Design review of the part built by this model. Coordinates are the model's own, in mm. A direction names the side the tool comes from. Coordinates: 2 decimals unless noted, no trailing zeros. Order: outer loops, then holes, each group sorted by start corner. A loop starts at its lowest first (then second) coordinate and runs counter-clockwise, first axis right, second up.
Autodesk Inventor part; units mm, degrees
ref_plane "YZ Plane" through (0, 0, 0) normal (1, 0, 0) x (0, 1, 0)
ref_plane "XZ Plane" through (0, 0, 0) normal (0, 1, 0) x (-1, 0, 0)
ref_plane "XY Plane" through (0, 0, 0) normal (0, 0, 1) x (1, 0, 0)
sketch "Sketch1" plane through (0, 0, 0) normal (0, 1, 0) x (-1, 0, 0)
  line L0 (-52.0419, 20) -> (-52.0419, -20)
  line L1 (52.0419, 20) -> (-52.0419, -20) construction
  line L2 (-52.0419, 20) -> (52.0419, -20) construction
  line L3 (305.5497, 112) -> (270.3665, 112)
  line L4 (270.3665, -112) -> (305.5497, -112)
  line L5 (305.5497, -112) -> (305.5497, 112)
  line L6 (305.5497, 112) -> (270.3665, -112) construction
  line L7 (270.3665, 112) -> (305.5497, -112) construction
  line L8 (270.3665, 20) -> (-52.0419, 20)
  line L9 (270.3665, 112) -> (270.3665, 20)
  line L10 (270.3665, -20) -> (270.3665, -112)
  line L11 (-52.0419, -20) -> (270.3665, -20)
  point P0 (0, 0)
  point P1 (287.9581, 0)
  point P2 (-52.0419, 0)
  dimension "d17" = 224
  dimension "d19" = 40
  dimension "d20" = 340
extrude "Extrusion1" add sketch "Sketch1" along normal blind 34
sketch "Sketch2" plane through (-305.5497, 0, 112) normal (0, 0, 1) x (1, 0, 0)
  circle A0 centre (17.5916, 16) radius 4.25
  line L0 (0, 0) -> (35.1832, 0)
  line L1 (0, 0) -> (0, 34)
  point P0 (305.5497, 0)
  point P1 (17.5916, 0)
  dimension "d2" = 8.5
  dimension "d3" = 16
sketch "Sketch3" plane through (52.0419, 0, 20) normal (1, 0, 0) x (0, 0, -1)
  circle A0 centre (20, 16) radius 4.25
  line L0 (0, 0) -> (40, 0)
  line L1 (40, 0) -> (40, 34)
  point P0 (20, 0)
  point P1 (20, 0)
  dimension "d4" = 8.5
  dimension "d5" = 16
sketch "Sketch4" plane through (-270.3665, 0, -112) normal (0, 0, -1) x (-1, 0, 0)
  circle A0 centre (17.5916, 16) radius 4.25
  line L0 (0, 0) -> (35.1832, 0)
  line L1 (0, 0) -> (0, 34)
  point P0 (-270.3665, 0)
  point P1 (17.5916, 0)
  dimension "d6" = 8.5
  dimension "d7" = 16
extrude "Extrusion2" cut sketch "Sketch4" against normal blind 10
extrude "Extrusion3" cut sketch "Sketch2" against normal blind 10
extrude "Extrusion4" cut sketch "Sketch3" against normal blind 10
properties part number "T"
1. For faces 4 (the cylindrical face through (47.11, 11.85, 0.92)), 5 (the flat face through (-111, 17, 20)), 6 (the cylindrical face through (-292.204, 16.187, 107.07)), list the 3-axis set-ups (+Z, -Z, +X, -X, +Y, -Y) from which the entire face can be reached by the end or side of a thin tool; tool diameter is ignored.
2. Add section B-B (z = -38.5). Give the boundary of the cut face in (x, y), and give its area (3 significant figures).
3. Insertion check: pin 1 (4 mm diameter, centred on x = -122, y = 24, fed in from +Z); pin 2 (17 mm diameter, centred on y = 9, z = -53, fed in from +X); pin 3 (10 mm diameter, centred on x = -117, y = 23.5, fed in from -Z). Each pin has a flat end and moves straight along its axis. Give the tip position at first contact, or say it passes through.
4. Add section A-A (y = 16). Give the boundary of the cut face in (x, z), and give its area (3 significant figures).
5. To check wall thickness, follow line 1 (Y direction, x = 46, z = 0); line 2 (Z direction, x = -9.5, y = 23); line 3 (X direction, y = 5, z = -80). State the ranges of each line that lie inside material, in increasing order.
6. Mouldability with a two-part tool opening along X and no side actions: class faces 1 (the flat face through (-107, 17, -20)), 2 (the flat face through (-288, 16, 102)), 3 (the flat face through (-270.366, 17, 67)) as pulls with the +X half, pulls with the -X half, needs draft (parallel to the pull), parting line crosses it, or undercut.
7. Add section C-C (x = -211). Give the boundary of the cut face in (y, z).
Solution:
1. face 4: +X
1. face 5: +Z, +X, +Y, -Y
1. face 6: +Z
2. outline: (-305.55, 0) - (-270.37, 0) - (-270.37, 34) - (-305.55, 34) - close
2. area: 1,200 mm2
3. pin 1: stops at z = 20
3. pin 2: stops at x = -270.37
3. pin 3: stops at z = -20
4. outline: (-305.55, -112) - (-292.21, -112) - (-292.21, -102) - (-283.71, -102) - (-283.71, -112) - (-270.37, -112) - (-270.37, -20) - (52.04, -20) - (52.04, -4.25) - (42.04, -4.25) - (42.04, 4.25) - (52.04, 4.25) - (52.04, 20) - (-270.37, 20) - (-270.37, 112) - (-283.71, 112) - (-283.71, 102) - (-292.21, 102) - (-292.21, 112) - (-305.55, 112) - close
4. area: 20,500 mm2
5. line 1: y = 0 to 11.75, 20.25 to 34
5. line 2: z = -20 to 20
5. line 3: x = -305.55 to -270.37
6. face 1: needs draft
6. face 2: undercut
6. face 3: pulls with the +X half
7. outline: (0, -20) - (34, -20) - (34, 20) - (0, 20) - close
